Verification items for this drawing (mm, ordinates from the low corner). Coordinates: 2 decimals unless noted, no trailing zeros. Write each loop counter-clockwise with the first axis right and the second up, starting at its lowest first coordinate (ties: lowest second). Pieces come first, ordered by that corner, then holes.
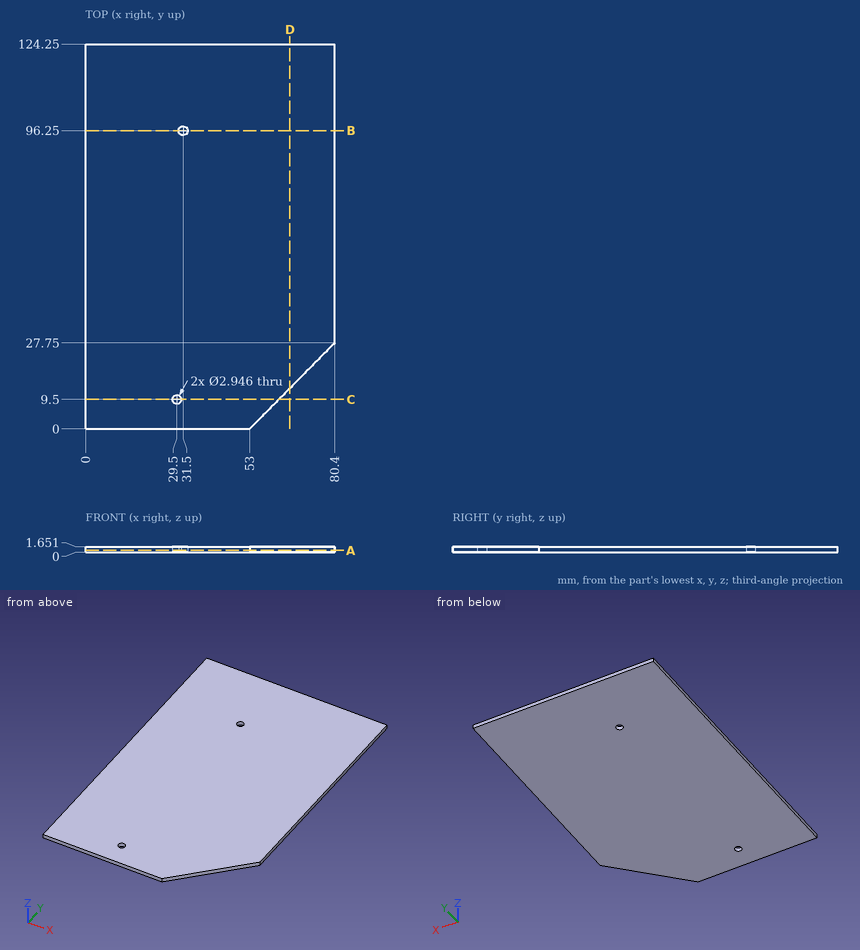
1. Sectioned sample at B-B, the plane y = 96.25. Record the boundary of the cut face in (x, z).
Computed values:
outline: (0, 0) - (30.03, 0) - (30.03, 1.65) - (0, 1.65) - close; (32.97, 0) - (80.4, 0) - (80.4, 1.65) - (32.97, 1.65) - close
2. Sectioned sample at A-A, the plane z = 0.5. Record the boundary of the cut face in (x, y), and give its area (3 significant figures).
Computed values:
outline: (0, 0) - (53, 0) - (80.4, 27.75) - (80.4, 124.25) - (0, 124.25) - close; hole circle Ø2.95 at (29.5, 9.5); hole circle Ø2.95 at (31.5, 96.25)
area: 9,600 mm2
3. Thickness scan on line 1 along Y through (x, z) = (29.5, 0.9); line 2 along X through (y, z) = (96.25, 0.4); line 3 along Y through (x, z) = (28.5, 0.6). Record the ranges inside material, lowest first.
Computed values:
line 1: y = 0 to 8.03, 10.97 to 124.25
line 2: x = 0 to 30.03, 32.97 to 80.4
line 3: y = 0 to 8.42, 10.58 to 124.25
4. Sectioned sample at C-C, the plane y = 9.5. Record the boundary of the cut face in (x, z).
Computed values:
outline: (0, 0) - (28.03, 0) - (28.03, 1.65) - (0, 1.65) - close; (30.97, 0) - (62.38, 0) - (62.38, 1.65) - (30.97, 1.65) - close
5. Sectioned sample at D-D, the plane x = 66. Record the boundary of the cut face in (y, z).
Computed values:
outline: (13.17, 0) - (124.25, 0) - (124.25, 1.65) - (13.17, 1.65) - close
